The model under review builds one solid part; all positions refer to its coordinate system, in mm. Face numbers are marked on the shaded views. A direction names the side the tool comes from. Round coordinates to 2 decimals unless told otherwise and drop trailing zeros. Order: outer loops, then holes, each group sorted by start corner. A loop starts at its lowest first (then second) coordinate and runs counter-clockwise, first axis right, second up. Notation, with made-up numbers: M 3.25,51 L 50.25,51 A10 ccw 50.25,65 Z; hole C -31,-3.5 d2. An arc over 180 degrees is marked long. Answer as a JSON object with one key per item and string values. Group by question number.
1) Consider section C-C, the plane x = -11.5. Write out the cut boundary in (y, z), then the cut area to 3 significant figures.
2) For the marked faces 1 and 2, list the 3-axis set-ups (+Z, -Z, +X, -X, +Y, -Y) from which the entire face can be reached by the end or side of a thin tool; tool diameter is ignored.
3) To check wall thickness, follow line 1 (Y direction, x = 13, z = 0.35); line 2 (Y direction, x = 15.5, z = 2.95); line 3 (X direction, y = 2.5, z = 3.4). State the ranges of each line that lie inside material, in increasing order.
4) Consider section A-A, the plane y = -22. Write out the cut boundary in (x, z).
5) Insertion check: pin 1 Ø1.2 at (x, y) = (-1, 28) entering from +Z; pin 2 Ø1 at (x, z) = (-6, 3) entering from -Y; pin 3 Ø1.6 at (x, z) = (6.5, 3) entering from +Y. Each pin has a flat end and moves straight along its axis. Give the tip position at first contact, or say it passes through.
6) Consider section B-B, the plane z = 0.95. Write out the cut boundary in (x, y), then the cut area to 3 significant figures.
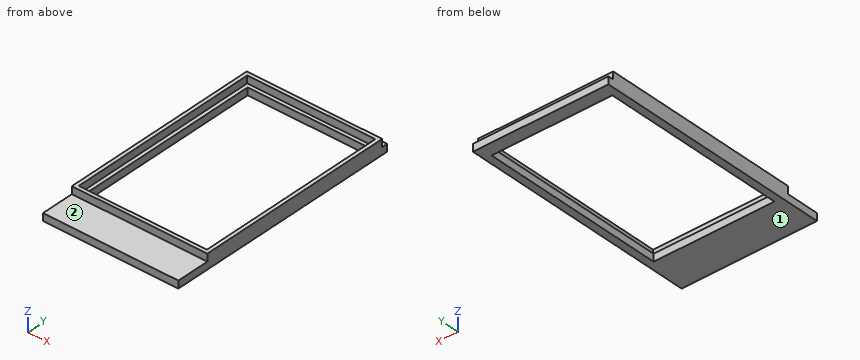
```python
from build123d import *

# Parameters (mm, degrees)
F0_W     = 36.8
F0_H     = 54.5
F0_W_2   = 34.8
F0_H_2   = 52.5
F0_H_3   = 1.5
F0_H_4   = 9
F0_W_3   = 32.8
F0_H_5   = 50.5
F1_DEPTH = 2
F2_DEPTH = 4


with BuildPart() as f1:
    # F0 (on Top) → F1 (new body)
    with BuildSketch(Plane.XY):
        Rectangle(F0_W, F0_H)
        Rectangle(F0_W_2, F0_H_2, mode=Mode.SUBTRACT)
        with Locations((0, 28)):
            Rectangle(F0_W, F0_H_3)
        with Locations((0, -31.75)):
            Rectangle(F0_W, F0_H_4)
        Rectangle(F0_W_2, F0_H_2)
        Rectangle(F0_W_3, F0_H_5, mode=Mode.SUBTRACT)
    extrude(amount=F1_DEPTH)

    # F0 (on Top) → F2 (join)
    with BuildSketch(Plane.XY):
        Rectangle(F0_W, F0_H)
        Rectangle(F0_W_2, F0_H_2, mode=Mode.SUBTRACT)
    extrude(amount=F2_DEPTH)


solid = f1.part
```
Results list:
{
 "1": {"outline": "M -36.25,0 L -25.25,0 L -25.25,2 L -26.25,2 L -26.25,4 L -27.25,4 L -27.25,2 L -36.25,2 Z; M 25.25,0 L 28.75,0 L 28.75,2 L 27.25,2 L 27.25,4 L 26.25,4 L 26.25,2 L 25.25,2 Z", "area": "33.0 mm^2"},
 "2": {"face 1": "-Z, +X, -X, +Y, -Y", "face 2": "+Z, +X, -X, -Y"},
 "3": {"line 1": "-36.25 to -25.25, 25.25 to 28.75", "line 2": "-27.25 to -26.25, 26.25 to 27.25", "line 3": "-18.4 to -17.4, 17.4 to 18.4"},
 "4": {"outline": "M -18.4,0 L -16.4,0 L -16.4,2 L -17.4,2 L -17.4,4 L -18.4,4 Z; M 16.4,0 L 18.4,0 L 18.4,4 L 17.4,4 L 17.4,2 L 16.4,2 Z"},
 "5": {"pin 1": "z = 2", "pin 2": "y = -27.25", "pin 3": "y = 27.25"},
 "6": {"outline": "M -18.4,-36.25 L 18.4,-36.25 L 18.4,28.75 L -18.4,28.75 Z; hole M -16.4,-25.25 L 16.4,-25.25 L 16.4,25.25 L -16.4,25.25 Z", "area": "736 mm^2"}
}
